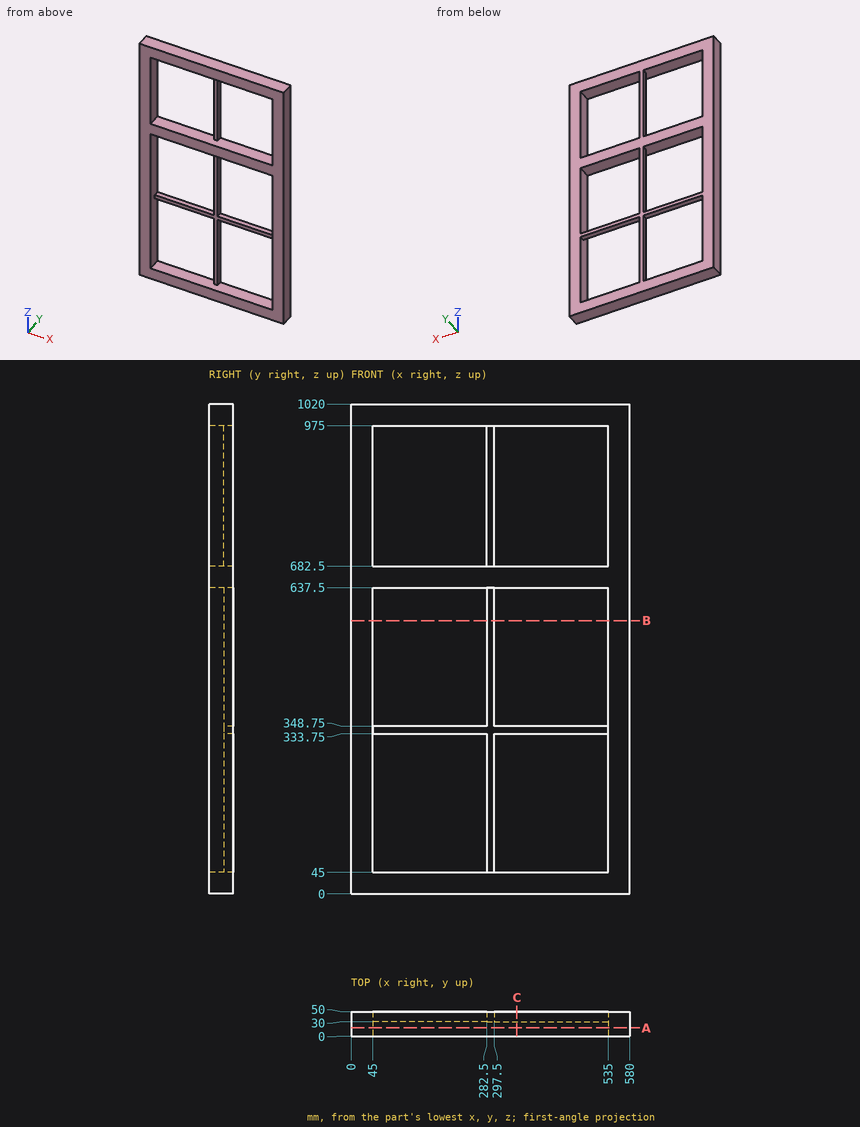
Can you work these out from the drawing? Everything is in mm from the part's minimum corner. Round coordinates to 2 decimals unless told otherwise and drop trailing zeros. Loops run counter-clockwise (first coordinate to the right, second up) from the corner with the lowest first, then second, coordinate; pieces in that order, holes last. Notation, with made-up numbers: (-30.75, -25) - (5.25, -25) arc R16 ccw to (5.25, -13) - close; hole circle Ø4 at (22.5, 60). An arc over 180 degrees is marked (long way). One line per question, with ' | ' between items. Start each with the question number.
Q1. Please list where these lines run through material, in increasing order: line 1 (X direction, y = 34.5, z = 248.5); line 2 (Z direction, x = 502.5, y = 7); line 3 (Z direction, x = 255, y = 48). Write a range as [from, to].
Q2. I want a section at A-A (y = 17). Write out the boundary of the cut face in (x, z).
Q3. I want a section at B-B (z = 569). Write out the boundary of the cut face in (x, y), then the cut area to 3 significant figures.
Q4. I want a section at C-C (x = 345). Write out the boundary of the cut face in (y, z), then the cut area to 3 significant figures.
Response values:
1) line 1: x = [0, 45], [282.5, 297.5], [535, 580] | line 2: z = [0, 45], [637.5, 682.5], [975, 1020] | line 3: z = [0, 45], [333.75, 348.75], [637.5, 682.5], [975, 1020]
2) outline: (0, 0) - (580, 0) - (580, 1020) - (0, 1020) - close; hole (45, 45) - (535, 45) - (535, 637.5) - (45, 637.5) - close; hole (45, 682.5) - (535, 682.5) - (535, 975) - (45, 975) - close
3) outline: (0, 0) - (45, 0) - (45, 50) - (0, 50) - close; (282.5, 30) - (297.5, 30) - (297.5, 50) - (282.5, 50) - close; (535, 0) - (580, 0) - (580, 50) - (535, 50) - close | area: 4,800 mm²
4) outline: (0, 0) - (50, 0) - (50, 45) - (0, 45) - close; (0, 637.5) - (50, 637.5) - (50, 682.5) - (0, 682.5) - close; (0, 975) - (50, 975) - (50, 1020) - (0, 1020) - close; (30, 333.75) - (50, 333.75) - (50, 348.75) - (30, 348.75) - close | area: 7,050 mm²
